from build123d import *

# Parameters (mm, degrees)
BOSS_EXTRUDE1_DEPTH = 29.5
BOSS_EXTRUDE2_DEPTH = 59
SKETCH3_W           = 1.4
SKETCH3_H           = 4.8
BOSS_EXTRUDE3_DEPTH = 3
FILLET1_R           = 0.5
SKETCH5_R           = 1.2
CUT_EXTRUDE1_DEPTH  = 13
SKETCH6_R           = 2.25
CUT_EXTRUDE2_DEPTH  = 5
FILLET2_R           = 0.2


with BuildPart() as part:
    # Sketch1 → Boss-Extrude1 (new body, symmetric)
    with BuildSketch(Plane.XY):
        Polygon((17.556624327, 0), (9.040707856, 14.75), (10.484083529, 14.75), (19, 0), (10.484083529, -14.75), (9.040707856, -14.75), align=None)
    extrude(amount=BOSS_EXTRUDE1_DEPTH, both=True)

    # Sketch2 → Boss-Extrude2 (add)
    with BuildSketch(Plane.XY.offset(29.5)):
        Polygon((17.556624327, 0), (14.5, 5.294228634), (14.5, -5.294228634), align=None)
    extrude(amount=-BOSS_EXTRUDE2_DEPTH)

    # Sketch3 → Boss-Extrude3 (add)
    with BuildSketch(Plane.XY.offset(29.5)):
        with Locations((15.85, 0)):
            Rectangle(SKETCH3_W, SKETCH3_H)
    extrude(amount=BOSS_EXTRUDE3_DEPTH)

    # Fillet1
    fillet1_edges = [part.edges().sort_by_distance(p)[0] for p in [
        (15.15, 0, 32.5),
        (15.85, -2.4, 32.5),
        (16.55, 0, 32.5),
        (15.85, 2.4, 32.5),
    ]]
    fillet(fillet1_edges, radius=FILLET1_R)

    # Sketch5 → Cut-Extrude1 (cut)
    with BuildSketch(Plane(origin=(20, 0, 0), x_dir=(0, 0, -1), z_dir=(1, 0, 0))):
        Circle(SKETCH5_R)
    extrude(amount=-CUT_EXTRUDE1_DEPTH, mode=Mode.SUBTRACT)

    # Sketch6 → Cut-Extrude2 (cut)
    with BuildSketch(Plane(origin=(20, 0, 0), x_dir=(0, 0, -1), z_dir=(1, 0, 0))):
        Circle(SKETCH6_R)
    extrude(amount=-CUT_EXTRUDE2_DEPTH, mode=Mode.SUBTRACT)

    # Fillet2
    fillet2_edges = [part.edges().sort_by_distance(p)[0] for p in [
        (15.15, 2.4, 30.75),
        (16.55, 2.4, 30.75),
        (16.55, -2.4, 30.75),
        (15.15, -2.4, 30.75),
        (16.373024454, -2.223024454, 32.381648008),
        (15.326975546, -2.223024454, 32.381648008),
        (16.373024454, 2.223024454, 32.381648008),
        (15.326975546, 2.223024454, 32.381648008),
    ]]
    fillet(fillet2_edges, radius=FILLET2_R)


solid = part.part
Source: CAD feature listing. Evaluate the final solid. Frame: model axes, mm. A direction names the side the tool comes from. Round coordinates to 2 decimals unless told otherwise and drop trailing zeros. Loops run counter-clockwise (first coordinate to the right, second up) from the corner with the lowest first, then second, coordinate; pieces in that order, holes last. Notation, with made-up numbers: (44, 42.25) - (93, 42.25) arc R12 ccw to (93, 57.25) - close; hole circle Ø2 at (7, 75). An arc over 180 degrees is marked (long way). Write item = value, one per line. Start each with the question number.
(1) Pull-direction query (Y, two-part tool) for faces 1 (the face through (16.584, 0.099, 2.248)), 2 (the face through (15, 0, -29.5)), 3 (the face through (14.802, -7.272, 0.413)); classes: +Y half, -Y half, draft (parallel to the pull), parting line (faces both ways), or undercut.
(2) Section query B-B, the plane z = 0. Output: boundary loops of the cut face in (x, y), plus the area to 3 significant figures.
(3) Set-up query: faces 4 (the face through (15.15, 0, 31)), 5 (the face through (14.68, 7.48, 0.41)), 6 (the face through (15, -1, -1)), 7 (the face through (16.55, 0, 31)), 8 (the face through (11.73, -10.09, 0.41)). Return all of +Z, -Z, +X, -X, +Y, -Y with unobstructed straight access to the full face (end or side cutting, diameter ignored); none if empty.
(4) Section query A-A, the plane x = 18.25. Output: boundary loops of the cut face in (y, z), plus the area to 3 significant figures.
(5) Ray query, line 1 along Z through (x, y) = (17.8, 0); line 2 along Z through (x, y) = (15.95, 0); line 3 along Y through (x, z) = (14, -20). Return the intervals inside material, ascending. Write a range as from..to.
(6) Pin query (flat end, axial travel): pin 1 (2.5 mm diameter, centred on y = 0, z = 0, fed in from -X); pin 2 (1 mm diameter, centred on y = -8.5, z = 7, fed in from +X); pin 3 (0.8 mm diameter, centred on y = 0, z = 31.5, fed in from -X). Return the tip coordinate at first contact, or that it passes through.
(7) Section query D-D, the plane x = 11.25. Output: boundary loops of the cut face in (y, z), plus the area to 3 significant figures.
(8) Section query C-C, the plane z = 24.5. Output: boundary loops of the cut face in (x, y), plus the area to 3 significant figures.
Conclusion:
q1.face_1 = undercut
q1.face_2 = draft
q1.face_3 = -Y half
q2.outline = (9.04, -14.75) - (10.48, -14.75) - (17.7, -2.25) - (15, -2.25) - (15, -1.2) - (14.5, -1.2) - (14.5, -5.29) - close; (9.04, 14.75) - (14.5, 5.29) - (14.5, 1.2) - (15, 1.2) - (15, 2.25) - (17.7, 2.25) - (10.48, 14.75) - close
q2.area = 42.5 mm2
q3.face_4 = +Z, -X, +Y, -Y
q3.face_5 = +Z, -Z, +X, +Y
q3.face_6 = +X
q3.face_7 = +Z, +X, +Y, -Y
q3.face_8 = +Z, -Z, -X
q4.outline = (-1.3, -29.5) - (1.3, -29.5) - (1.3, -1.84) arc R2.25 cw to (-1.3, -1.84) - close; (-1.3, 1.84) arc R2.25 cw to (1.3, 1.84) - (1.3, 29.5) - (-1.3, 29.5) - close
q4.area = 142 mm2
q5.line_1 = -29.5..-2.25, 2.25..29.5
q5.line_2 = -29.5..-2.25, 2.25..32.5
q5.line_3 = -8.66..-6.16, 6.16..8.66
q6.pin_1 = 14.5
q6.pin_2 = 14.38
q6.pin_3 = 15.15
q7.outline = (-13.42, -29.5) - (-10.92, -29.5) - (-10.92, 29.5) - (-13.42, 29.5) - close; (10.92, -29.5) - (13.42, -29.5) - (13.42, 29.5) - (10.92, 29.5) - close
q7.area = 295 mm2
q8.outline = (9.04, -14.75) - (10.48, -14.75) - (19, 0) - (10.48, 14.75) - (9.04, 14.75) - (14.5, 5.29) - (14.5, -5.29) - close
q8.area = 58.8 mm2
